Here's how the part is built. I have some questions about the finished solid (model axes, mm). A direction names the side the tool comes from. Coordinates: 2 decimals unless noted, no trailing zeros. Write each loop counter-clockwise with the first axis right and the second up, starting at its lowest first coordinate (ties: lowest second). Pieces come first, ordered by that corner, then holes.
Item 1: I want a section at A-A (z = 1.05). Count the separate pieces of the cut face and the enclosed holes in it, and give its area (3 significant figures).
Item 2: I want a section at B-B (y = 19.5). Please give me the cut outline in (x, z), and give its area (3 significant figures).
Item 3: Please list where these lines run through material, in increasing order: line 1 (X direction, y = 6, z = 1.75); line 2 (Z direction, x = 26.5, y = -20); line 3 (X direction, y = 14, z = 0.6).
Item 4: I'm going to push flat-ended pins straight in: P1, Ø3.5, axis at x = 53, y = 3, coming from the +Z side; P2, Ø1.5, axis at y = -16, z = 1.5, coming from the -X side; P3, Ø0.6, axis at y = -30, z = -1.5, coming from the -X side; P4, Ø1, axis at y = -26, z = -0.5, coming from the +X side. Where does each tip first touch, or does it pass through?
Item 5: I want a section at C-C (x = 35). Please give me the cut outline in (y, z), and give its area (3 significant figures).
Item 6: For faces 4 (the face through (-54.99, -8.91, 0.99)), 5 (the face through (-63, -21.926, -1)), 6 (the face through (-74, 2, 0)), which set-ups out of +Z, -Z, +X, -X, +Y, -Y let a thin tool reach every point of the face, with its end or its side?
Item 7: If we mould it in two halves opening along Y, with no side actions, what happens to faces 1 (the face through (-39.99, -8.91, 0.99)), 2 (the face through (43, 26.074, -1)), 3 (the face through (-42, -10, 2))? For each: pulls with the +Y half, pulls with the -Y half, needs draft (parallel to the pull), parting line crosses it, or undercut.
Item 8: I want a section at D-D (x = -8.5). Please give me the cut outline in (y, z), and give its area (3 significant figures).
from build123d import *

# Parameters (mm, degrees)
F0_R     = 2.5
F0_W     = 20
F0_H     = 48
F0_W_2   = 3
F0_W_3   = 2
F1_DEPTH = 2
F2_DEPTH = 2
F3_D     = 3.3
F3_DEPTH = 2.001
F4_D     = 3.3


# Not quite as in the source:
# - a feature names something its author has since deleted; it is built from what else it names


with BuildPart() as f1:
    # F0 (on Top) → F1 (new body)
    with BuildSketch(Plane.XY):
        Polygon((-17.7864517868, 26.073888598), (-50.0104304813, 26.073888598), (-50.0104304813, -21.926111402), (-17.7864517868, -21.926111402), (19.2135482132, -21.926111402), (29.9895695187, -21.926111402), (29.9895695187, 26.073888598), (19.2135482132, 26.073888598), align=None)
        with Locations((-42.2986224294, -7.9553306252)):
            Circle(F0_R, mode=Mode.SUBTRACT)
        with Locations((-42.2986224294, 13.5446693748)):
            Circle(F0_R, mode=Mode.SUBTRACT)
        Polygon((-50.0104304813, -21.926111402), (-50.0104304813, 26.073888598), (-54.2864517868, 26.073888598), (-70.0104304813, 26.073888598), (-70.0104304813, -21.926111402), (-54.2864517868, -21.926111402), align=None)
        with Locations((-57.2986224294, -7.9553306252)):
            Circle(F0_R, mode=Mode.SUBTRACT)
        with Locations((-57.2986224294, 13.5446693748)):
            Circle(F0_R, mode=Mode.SUBTRACT)
        with Locations((39.9895695187, 2.073888598)):
            Rectangle(F0_W, F0_H)
        Polygon((29.9895695187, 37.073888598), (-50.0104304813, 37.073888598), (-50.0104304813, 26.073888598), (-17.7864517868, 26.073888598), (19.2135482132, 26.073888598), (29.9895695187, 26.073888598), align=None)
        Polygon((-17.7864517868, -21.926111402), (-50.0104304813, -21.926111402), (-50.0104304813, -32.926111402), (29.9895695187, -32.926111402), (29.9895695187, -21.926111402), (19.2135482132, -21.926111402), align=None)
        with Locations((-73.5104304813, 2.073888598)):
            Rectangle(F0_W_2, F0_H)
        with Locations((53.4895695187, 2.073888598)):
            Rectangle(F0_W_2, F0_H)
        with Locations((-71.0104304813, 2.073888598)):
            Rectangle(F0_W_3, F0_H)
        with Locations((50.9895695187, 2.073888598)):
            Rectangle(F0_W_3, F0_H)
        with Locations((-42.2986224294, 13.5446693748)):
            Circle(F0_R)
        with Locations((-42.2986224294, -7.9553306252)):
            Circle(F0_R)
        with Locations((-57.2986224294, -7.9553306252)):
            Circle(F0_R)
        with Locations((-57.2986224294, 13.5446693748)):
            Circle(F0_R)
    extrude(amount=-F1_DEPTH)

    # F0 (on Top) → F2 (join)
    with BuildSketch(Plane.XY):
        with Locations((-71.0104304813, 2.073888598)):
            Rectangle(F0_W_3, F0_H)
        with Locations((50.9895695187, 2.073888598)):
            Rectangle(F0_W_3, F0_H)
        with Locations((-57.2986224294, 13.5446693748)):
            Circle(F0_R)
        with Locations((-42.2986224294, 13.5446693748)):
            Circle(F0_R)
        with Locations((-42.2986224294, -7.9553306252)):
            Circle(F0_R)
        with Locations((-57.2986224294, -7.9553306252)):
            Circle(F0_R)
    extrude(amount=F2_DEPTH)

    # F3 (through all, one way)
    with BuildSketch(Plane.XY):
        with Locations((-23.5104304813, 3.073888598), (3.4895695187, 3.073888598), (3.4895695187, 34.073888598), (-23.5104304813, 34.073888598), (-57.2986224294, 13.5446693748), (-42.2986224294, 13.5446693748), (-42.2986224294, -7.9553306252), (-57.2986224294, -7.9553306252)):
            Circle(F3_D / 2)
    extrude(amount=-F3_DEPTH, mode=Mode.SUBTRACT)

    # F4 (through all)
    with Locations(Plane(origin=(0, 0, 0), x_dir=(1, 0, 0), z_dir=(0, 0, -1))):
        with Locations((-57.2986224294, -13.5446693748), (-57.2986224294, 7.9553306252), (-42.2986224294, -13.5446693748), (-42.2986224294, 7.9553306252)):
            Hole(F4_D / 2)


solid = f1.part
Answer:
1. separate pieces: 6
1. enclosed holes: 4
1. area: 236 mm2
2. outline: (-75.01, -2) - (54.99, -2) - (54.99, 0) - (51.99, 0) - (51.99, 2) - (49.99, 2) - (49.99, 0) - (-70.01, 0) - (-70.01, 2) - (-72.01, 2) - (-72.01, 0) - (-75.01, 0) - close
2. area: 268 mm2
3. line 1: x = -72.01 to -70.01, 49.99 to 51.99
3. line 2: z = -2 to 0
3. line 3: x = -72.01 to -70.01, -59.76 to -58.88, -55.71 to -54.84, -44.76 to -43.88, -40.71 to -39.84, 49.99 to 51.99
4. P1: stops at z = 2
4. P2: stops at x = -72.01
4. P3: stops at x = -50.01
4. P4: stops at x = 29.99
5. outline: (-21.93, -2) - (26.07, -2) - (26.07, 0) - (-21.93, 0) - close
5. area: 96.0 mm2
6. face 4: +Z
6. face 5: +Z, -Z, -X, -Y
6. face 6: +Z, -X, +Y, -Y
7. face 1: undercut
7. face 2: pulls with the +Y half
7. face 3: needs draft
8. outline: (-32.93, -2) - (37.07, -2) - (37.07, 0) - (-32.93, 0) - close
8. area: 140 mm2
